Read the model definition and answer for the solid it produces. Units are mm, in the model's axes. Face numbers are marked on the shaded views. A direction names the side the tool comes from. Coordinates: 2 decimals unless noted, no trailing zeros. Order: outer loops, then holes, each group sorted by start corner. A loop starts at its lowest first (then second) coordinate and runs counter-clockwise, first axis right, second up. Notation, with made-up numbers: M -21.75,55 L -17.75,55 A25 ccw -17.75,91 Z; hole C 17.5,-36 d2. An arc over 180 degrees is marked long. Use a Markdown table: item, result. Add a question column.
1) The mould has two halves that part along Y. Classify the marked faces 5, 6 and 7: released by +Y, released by -Y, zero draft, split by the parting line, or undercut.
2) Find section A-A on x = -4.5. Write down the section's boundary in (y, z).
3) Find the intervals of material crossed by probe 1 along X at (y, z) = (0, 7); probe 2 along X at (y, z) = (9.25, 5.75); probe 3 along Z at (x, y) = (6.5, 6.75), in increasing order. Write a range as [from, to].
4) Each of these flat-tipped pins is pushed along its axis until it touches: pin 1 Ø1.5 at (y, z) = (5.5, 7.5) entering from +X; pin 2 Ø1 at (x, z) = (-11.5, 4.5) entering from +Y; pin 3 Ø2.5 at (y, z) = (-2.5, 6) entering from +X. Where does it stop, or does it pass through?
5) For the marked faces 1, 2, 3 and 4, determine the directions among +Z, -Z, +X, -X, +Y, -Y from which every point of the face is accessible in a straight line to the end or side of a thin tool.
6) Find section B-B on z = 6.5. Count the separate pieces of the cut face and the enclosed holes in it, plus the area to 3 significant figures.
7) Find section D-D on x = 19. Write down the section's boundary in (y, z), plus the area to 3 significant figures.
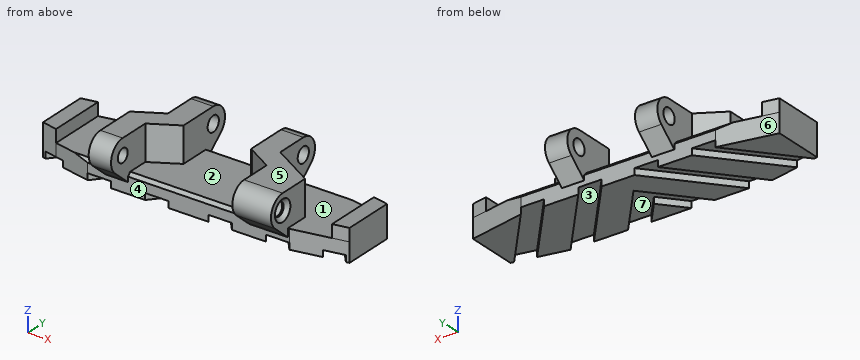
from build123d import *
from OCP.BRepAlgoAPI import BRepAlgoAPI_Cut
from OCP.TopTools import TopTools_ListOfShape

# Parameters (mm, degrees)
BOSS_EXTRUDE1_DEPTH    = 2.99974
BOSS_EXTRUDE2_DEPTH    = 5.00126
BOSS_EXTRUDE3_DEPTH    = 3.50012
CIRPATTERN1_COUNT      = 2
BOSS_EXTRUDE4_REACH    = 30.871
CUT_EXTRUDE1_DEPTH     = 5.5
CUT_EXTRUDE2_DEPTH     = 1.00076
MIRROR2_START          = -12.999258093
MIRROR2_DEPTH          = 7.70128
MIRROR2_START_2        = 2.99974
MIRROR2_2_DEPTH        = 5.5
MIRROR2_3_OUTLINE_W    = 4.20116
MIRROR2_3_OUTLINE_H    = 4.60831964
MIRROR2_3_OUTLINE_H_2  = 4.995876312
MIRROR2_3_DEPTH        = 2.99974
MIRROR2_4_DEPTH        = 5.5
SKETCH9_R              = 1.05
OUTSIDE_HOLES_DEPTH    = 41.329539227
SKETCH10_R             = 1.2
INSIDE_HOLES_DEPTH     = 37.513584997
BOSS_EXTRUDE5_START    = 2.54
SKETCH12_R             = 1.05
BOSS_EXTRUDE5_DEPTH    = 2.54
HEAD_POCKET_DEPTH      = 1.7
HEAD_POCKET_DEPTH_BACK = 0.7
SKETCH11_R             = 1.45
CHAMFER1_SIZE          = 0.6
CORNER_CUT_DEPTH       = 5.5
CHAMFER2_SIZE          = 0.5


with BuildPart() as part:
    # Sketch1 → Boss-Extrude1 (new body)
    with BuildSketch(Plane(origin=(0, 0, 0), x_dir=(-1, 0, 0), z_dir=(0, 0, -1))):
        Polygon((23.999998093, 0.250000321), (23.999998093, 8.25), (15.229382515, 10.004123688), (-15.229382515, 10.004123688), (-23.999998093, 8.25), (-23.999998093, 0.25), (-15.791597366, -1.39168036), (15.791597366, -1.39168036), align=None)
    extrude(amount=-BOSS_EXTRUDE1_DEPTH)

    # Sketch2 → Boss-Extrude2 (add)
    with BuildSketch(Plane(origin=(0, 0, 0), x_dir=(-1, 0, 0), z_dir=(0, 0, -1))):
        Polygon((21.599998474, -0.230000138), (21.599998474, 8.729999542), (23.999998093, 8.25), (23.999998093, 0.249999762), align=None)
        Polygon((-23.999998093, 0.249999762), (-23.999998093, 8.25), (-21.599998474, 8.729999542), (-21.599998474, -0.230000138), align=None)
    extrude(amount=-BOSS_EXTRUDE2_DEPTH)

    # Sketch3 → Boss-Extrude3 (add)
    with BuildSketch(Plane(origin=(12.999258093, 0, 0), x_dir=(0, 0, -1), z_dir=(1, 0, 0))):
        with BuildLine():
            Line((-2.99974, 4.117571831), (-8.49974, 4.117571354))
            Line((-8.49974, 4.117571354), (-8.49974, -2.500000222))
            ThreePointArc((-8.49974, -2.500000222), (-6.87834524, -4.840080872), (-4.117836275, -4.144028668))
            Line((-4.117836275, -4.144028668), (-1.714206095, -1.39168036))
            Line((-1.714206095, -1.39168036), (-2.99974, -1.39168036))
            Line((-2.99974, -1.39168036), (-2.99974, 4.117571831))
        make_face()
    boss_extrude3 = extrude(amount=-BOSS_EXTRUDE3_DEPTH)

    # CirPattern1: Boss-Extrude3 ×2 about axis
    cirpattern1_axis = Axis((9.148618093, 4.306221664, 0), (0, 0, 1))
    for i in range(1, CIRPATTERN1_COUNT):
        add(boss_extrude3.rotate(cirpattern1_axis, i * 360 / CIRPATTERN1_COUNT))

    # Sketch4 → Boss-Extrude4 (add, up to next)
    with BuildSketch(Plane.XY.offset(8.49974), mode=Mode.PRIVATE) as boss_extrude4_sk1:
        Polygon((8.799999237, 6.184122562), (12.999999024, 3.759251555), (9.499999024, 2.315876444), (5.299999237, 4.740747452), align=None)
    boss_extrude4_tool1 = extrude(boss_extrude4_sk1.sketch, amount=-BOSS_EXTRUDE4_REACH, mode=Mode.PRIVATE) - part.part
    add(boss_extrude4_tool1.solids().sort_by_distance((9.149999, 4.25, 8.49974))[0])


with BuildPart() as cut_extrude1_tool:
    # Sketch5 → Cut-Extrude1 (new body)
    with BuildSketch(Plane.XY.offset(8.49974)):
        Polygon((12.999999024, 3.759251555), (12.999258093, 4.117571354), (12.379370927, 4.117571354), align=None)
        Polygon((5.725868057, 4.494871974), (5.297978093, 4.494871974), (5.297978093, 4.74191436), align=None)
    extrude(amount=-CUT_EXTRUDE1_DEPTH)


with BuildPart() as part_1:
    add(part.part)

    # Cut-Extrude1: cut by cut_extrude1_tool, with a tolerance
    cut_extrude1_stock = TopTools_ListOfShape()
    cut_extrude1_stock.Append(part_1.part.wrapped)
    cut_extrude1_tools = TopTools_ListOfShape()
    cut_extrude1_tools.Append(cut_extrude1_tool.part.wrapped)
    cut_extrude1_cut = BRepAlgoAPI_Cut()
    cut_extrude1_cut.SetArguments(cut_extrude1_stock)
    cut_extrude1_cut.SetTools(cut_extrude1_tools)
    cut_extrude1_cut.SetFuzzyValue(0.00001)
    cut_extrude1_cut.Build()
    add(Compound.cast(cut_extrude1_cut.Shape()).solids(), mode=Mode.REPLACE)


with BuildPart() as cut_extrude2_tool:
    # Sketch6 → Cut-Extrude2 (new body)
    with BuildSketch(Plane(origin=(0, 0, 0), x_dir=(-1, 0, 0), z_dir=(0, 0, -1))):
        Polygon((20.368379593, -0.476323605), (11.367927551, 10.25), (15.229382515, 10.004123688), (23.498262405, 0.149653077), align=None)
        Polygon((2.36792779, 10.25), (12.437123299, -1.75), (15.791597366, -1.39168036), (6.023067951, 10.25), align=None)
        Polygon((0, 6.702231407), (7.092263699, -1.75), (3.437123299, -1.75), (0, 2.346204281), (-3.437123299, -1.75), (-7.092263699, -1.75), align=None)
        Polygon((-15.791597366, -1.39168036), (-6.023067951, 10.25), (-2.36792779, 10.25), (-12.437123299, -1.75), align=None)
        Polygon((-11.367927551, 10.25), (-20.368379593, -0.476323605), (-23.498262405, 0.149653077), (-15.229382515, 10.004123688), align=None)
    extrude(amount=-CUT_EXTRUDE2_DEPTH)


with BuildPart() as part_2:
    add(part_1.part)

    # Cut-Extrude2: cut by cut_extrude2_tool, with a tolerance
    cut_extrude2_stock = TopTools_ListOfShape()
    cut_extrude2_stock.Append(part_2.part.wrapped)
    cut_extrude2_tools = TopTools_ListOfShape()
    cut_extrude2_tools.Append(cut_extrude2_tool.part.wrapped)
    cut_extrude2_cut = BRepAlgoAPI_Cut()
    cut_extrude2_cut.SetArguments(cut_extrude2_stock)
    cut_extrude2_cut.SetTools(cut_extrude2_tools)
    cut_extrude2_cut.SetFuzzyValue(0.00001)
    cut_extrude2_cut.Build()
    add(Compound.cast(cut_extrude2_cut.Shape()).solids(), mode=Mode.REPLACE)

    # Mirror2: read off the stored shape, not the designer's step
    # Mirror2 outline → Mirror2 (add)
    with BuildSketch(Plane.YZ.offset(MIRROR2_START)):
        with BuildLine():
            Line((11.11244355, 8.49974), (-2.500000222, 8.49974))
            ThreePointArc((-2.500000222, 8.49974), (-4.840080872, 6.87834524), (-4.144028668, 4.117836275))
            Line((-4.144028668, 4.117836275), (-1.39168036, 1.714206095))
            Line((-1.39168036, 1.714206095), (-1.39168036, 2.99974))
            Line((-1.39168036, 2.99974), (10.004123688, 2.99974))
            Line((10.004123688, 2.99974), (10.004123688, 1.714206095))
            Line((10.004123688, 1.714206095), (12.756471996, 4.117836275))
            ThreePointArc((12.756471996, 4.117836275), (13.4525242, 6.87834524), (11.11244355, 8.49974))
        make_face()
    extrude(amount=MIRROR2_DEPTH)

    # Mirror2 2 outline → Mirror2 2 (cut)
    with BuildSketch(Plane.XY.offset(MIRROR2_START_2)):
        Polygon((-5.297978093, 4.74191436), (-9.499138093, 2.316373503), (-9.499138093, -6), (-5.297978093, -6), align=None)
        Polygon((-12.999258093, 3.759679332), (-8.799999237, 6.184122562), (-8.798098093, 6.183338544), (-8.798098093, 15), (-12.999258093, 15), align=None)
    extrude(amount=MIRROR2_2_DEPTH, mode=Mode.SUBTRACT)

    # Mirror2 3 outline → Mirror2 3 (cut)
    with BuildSketch(Plane.XY):
        with Locations((-7.398558093, -3.69584018)):
            Rectangle(MIRROR2_3_OUTLINE_W, MIRROR2_3_OUTLINE_H)
        with Locations((-10.898678093, 12.502061844)):
            Rectangle(MIRROR2_3_OUTLINE_W, MIRROR2_3_OUTLINE_H_2)
    extrude(amount=MIRROR2_3_DEPTH, mode=Mode.SUBTRACT)

    # Mirror2 4 outline → Mirror2 4 (add)
    with BuildSketch(Plane.XY.offset(MIRROR2_START_2)):
        Polygon((-12.999999024, 3.759251555), (-12.999258093, 3.758946), (-12.999258093, 3.759679332), align=None)
    extrude(amount=MIRROR2_4_DEPTH)

    # Sketch9 → Outside_Holes (cut, through all)
    with BuildSketch(Plane(origin=(12.999258093, 0, 0), x_dir=(0, 0, -1), z_dir=(1, 0, 0))):
        with Locations((-6.00038, -2.500000222)):
            Circle(SKETCH9_R)
    extrude(amount=-OUTSIDE_HOLES_DEPTH, mode=Mode.SUBTRACT)

    # Sketch10 → Inside_Holes (cut, through all)
    with BuildSketch(Plane(origin=(8.798098093, 0, 0), x_dir=(0, 0, -1), z_dir=(1, 0, 0))):
        with Locations((-6.00038, 11.11244355)):
            Circle(SKETCH10_R)
    extrude(amount=-INSIDE_HOLES_DEPTH, mode=Mode.SUBTRACT)

    # Sketch12 → Boss-Extrude5 (add)
    with BuildSketch(Plane(origin=(12.999258093, 0, 0), x_dir=(0, 0, -1), z_dir=(1, 0, 0)).offset(BOSS_EXTRUDE5_START)):
        with BuildLine():
            Line((-2.99974, 3.758946), (-8.49974, 3.758946))
            Line((-8.49974, 3.758946), (-8.49974, -2.500000222))
            ThreePointArc((-8.49974, -2.500000222), (-6.87834524, -4.840080872), (-4.117836275, -4.144028668))
            Line((-4.117836275, -4.144028668), (-1.714206095, -1.39168036))
            Line((-1.714206095, -1.39168036), (-2.99974, -1.39168036))
            Line((-2.99974, -1.39168036), (-2.99974, 3.758946))
        make_face()
        with Locations((-6.00038, -2.500000222)):
            Circle(SKETCH12_R, mode=Mode.SUBTRACT)
    extrude(amount=-BOSS_EXTRUDE5_DEPTH)

    # Sketch11 → Head_Pocket (cut, two sides: drawn at the far end of the back side and taken through both)
    with BuildSketch(Plane(origin=(12.999258093, 0, 0), x_dir=(0, 0, -1), z_dir=(1, 0, 0)).offset(-HEAD_POCKET_DEPTH_BACK)):
        with Locations((-6.00038, -2.500000222)):
            Circle(SKETCH11_R)
    extrude(amount=HEAD_POCKET_DEPTH + HEAD_POCKET_DEPTH_BACK, mode=Mode.SUBTRACT)

    # Chamfer1
    chamfer1_edges = [part_2.edges().sort_by_distance(p)[0] for p in [
        (15.539258093, -2.500000222, 7.05038),
    ]]
    chamfer(chamfer1_edges, length=CHAMFER1_SIZE)

    # Sketch13 → Corner_Cut (cut)
    with BuildSketch(Plane.XY.offset(8.49974)):
        Polygon((15.539258093, 3.758946), (15.539258093, 2.292476317), (12.999258093, 3.758946), align=None)
    extrude(amount=-CORNER_CUT_DEPTH, mode=Mode.SUBTRACT)

    # Chamfer2
    chamfer2_edges = [part_2.edges().sort_by_distance(p)[0] for p in [
        (-10.898678093, 10.004123688, 2.99974),
        (-14.39542773, -1.39168036, 2.99974),
        (0, 10.004123688, 2.99974),
        (2.10058, -1.39168036, 2.99974),
        (12.013740304, 10.004123688, 2.99974),
    ]]
    chamfer(chamfer2_edges, length=CHAMFER2_SIZE)


solid = part_2.part
Check result:
| question | item | result |
|---|---|---|
| 1 | face 5 | zero draft |
| 1 | face 6 | released by +Y |
| 1 | face 7 | undercut |
| 2 | outline | M -1.39,1 L 1.34,1 L 1.34,0 L 7.71,0 L 7.71,1 L 10,1 L 10,2.5 L 9.5,3 L -0.89,3 L -1.39,2.5 Z |
| 3 | probe 1 | x = [-13, -9.5], [9.5, 15.54] |
| 3 | probe 2 | x = [-8.8, -5.3], [5.3, 8.8] |
| 3 | probe 3 | z = [1, 8.5] |
| 4 | pin 1 | stops at x = 11.28 |
| 4 | pin 2 | stops at y = 4.91 |
| 4 | pin 3 | stops at x = 15.14 |
| 5 | face 1 | +Z, +Y |
| 5 | face 2 | +Z, -Y |
| 5 | face 3 | -Z |
| 5 | face 4 | -Z, -Y |
| 6 | separate pieces | 6 |
| 6 | enclosed holes | 0 |
| 6 | area | 127 mm2 |
| 7 | outline | M -0.75,0 L 1.15,0 L 1.15,1 L 5.51,1 L 5.51,0 L 9.25,0 L 9.25,3 L -0.75,3 Z |
| 7 | area | 25.6 mm2 |
